Build history of the part. All positions in model axes, mm. Face numbers are marked on the shaded views. A direction names the side the tool comes from. Give positions to 0.01 mm unless a question says otherwise; leave off trailing zeros. Order: outer loops, then holes, each group sorted by start corner. A loop starts at its lowest first (then second) coordinate and runs counter-clockwise, first axis right, second up. Notation, with made-up numbers: (48, -38.75) -> (74, -38.75) arc R28 cw to (74, -17.75) -> close; hole circle Ø5 at (-26, 43). An arc over 180 degrees is marked (long way). One line per item, written item: value. Start each with the question number.
(1) Saw through at D-D on y = 4. Give the cut face in (x, z) (3 decimals).
(2) Saw through at A-A on y = -2. Give the cut face in (x, z) (3 decimals), plus the area to 3 significant figures.
(3) Saw through at B-B on y = 11. Give the cut face in (x, z) (3 decimals), plus the area to 3 significant figures.
(4) Two-plate mould, pull along X, no slides. Class the marked faces 1, 2 and 3: +X half, -X half, draft (parallel to the pull), parting line (faces both ways), or undercut.
(5) Saw through at C-C on x = -1.5. Give the cut face in (y, z) (3 decimals).
(6) Which spindle directions (+Z, -Z, +X, -X, +Y, -Y) get a long thin tool onto all of the face, cutting with end or side? Do the marked faces 4, 5, 6 and 7. Say none if no direction does.
(7) Pin check, flat tips, straight feed: pin 1 (1.3 mm diameter, centred on y = 23.5, z = 0.5, fed in from -X); pin 2 (3 mm diameter, centred on y = 18.5, z = 1.5, fed in from +X); pin 3 (3 mm diameter, centred on x = 13, z = 0, fed in from -Y); pin 4 (2.5 mm diameter, centred on x = -1, y = 11, fed in from +Z). Stop position of each tip, or through.
(8) Probe line 1 (X direction, y = -3.5, z = -1); line 2 (Z direction, x = 9.6, y = -6) (3 decimals); line 3 (Y direction, x = 13, z = 0). List the from-to ranges inside material, lowest first.
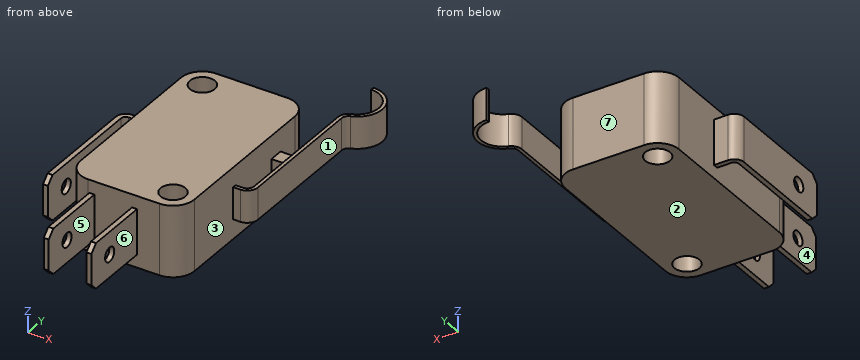
```python
from build123d import *

# Parameters (mm, degrees)
ESBO_O1_W             = 16
ESBO_O1_H             = 28
EXTRUS_O1_DEPTH       = 5
FILETE1_R             = 3
ESBO_O2_R             = 1.75
CORTE_EXTRUS_O1_DEPTH = 34.763886032
FLANGE_BASE1_START    = -2.25
FLANGE_BASE1_DEPTH    = 4.5
EXTRUS_O2_DEPTH       = 1.75
EXTRUS_O_FINA1_DEPTH  = 3.175
ESBO_O6_4_W           = 0.7
ESBO_O6_4_H           = 10
EXTRUS_O_FINA2_DEPTH  = 3.175
ESBO_O6_5_W           = 0.7
ESBO_O6_5_H           = 10
EXTRUS_O_FINA3_DEPTH  = 3.175
CHANFRO1_SIZE         = 1
ESBO_O7_R             = 1
CORTE_EXTRUS_O8_DEPTH = 3.35
ESBO_O7_6_R           = 1
CORTE_EXTRUS_O9_DEPTH = 47.597558949


# Read off the part's stored shape, not the designer's step: Flange-base1
with BuildPart() as part:
    # Esbo_o1 → Extrus_o1 (new, symmetric)
    with BuildSketch(Plane.XY):
        with Locations((8, 14)):
            Rectangle(ESBO_O1_W, ESBO_O1_H)
    extrude(amount=EXTRUS_O1_DEPTH, both=True)

    # Filete1
    filete1_edges = [part.edges().sort_by_distance(p)[0] for p in [
        (0, 28, 0),
        (16, 28, 0),
        (16, 0, 0),
        (0, 0, 0),
    ]]
    fillet(filete1_edges, radius=FILETE1_R)

    # Esbo_o2 → Corte-extrus_o1 (cut, through all)
    with BuildSketch(Plane.XY.offset(5)):
        with Locations((3, 25)):
            Circle(ESBO_O2_R)
        with Locations((13, 3)):
            Circle(ESBO_O2_R)
    extrude(amount=-CORTE_EXTRUS_O1_DEPTH, mode=Mode.SUBTRACT)



with BuildPart() as body_2:
    # Flange-base1 outline → Flange-base1 (new body)
    with BuildSketch(Plane.XY.offset(FLANGE_BASE1_START)):
        with BuildLine():
            ThreePointArc((19.166666667, 32.300168354), (21.449594959, 36.191856925), (18, 39.1))
            Line((18, 39.1), (18, 38.6))
            ThreePointArc((18, 38.6), (20.956795679, 36.107305936), (19, 32.771572875))
            ThreePointArc((19, 32.771572875), (18.275255129, 32.223384717), (18, 31.357359313))
            Line((18, 31.357359313), (18, 13))
            ThreePointArc((18, 13), (17.707106781, 12.292893219), (17, 12))
            Line((17, 12), (16, 12))
            Line((16, 12), (16, 11.5))
            Line((16, 11.5), (17, 11.5))
            ThreePointArc((17, 11.5), (18.060660172, 11.939339828), (18.5, 13))
            Line((18.5, 13), (18.5, 31.357359313))
            ThreePointArc((18.5, 31.357359313), (18.683503419, 31.934709582), (19.166666667, 32.300168354))
        make_face()
    extrude(amount=FLANGE_BASE1_DEPTH)


with BuildPart() as part_1:
    add(part.part)

    add(body_2.part)  # Extrus_o2 merges body 2
    # Esbo_o5 → Extrus_o2 (add, symmetric)
    with BuildSketch(Plane.XY):
        with BuildLine():
            Line((16, 21.874244368), (17.5, 21.874244368))
            ThreePointArc((17.5, 21.874244368), (17.853553391, 21.727797759), (18, 21.374244368))
            Line((18, 21.374244368), (18, 20.374244368))
            ThreePointArc((18, 20.374244368), (17.853553391, 20.020690978), (17.5, 19.874244368))
            Line((17.5, 19.874244368), (16, 19.874244368))
            Line((16, 19.874244368), (16, 21.874244368))
        make_face()
    extrude(amount=EXTRUS_O2_DEPTH, both=True)

    # Esbo_o6 → Extrus_o-Fina1 (add, symmetric)
    with BuildSketch(Plane.XY):
        with BuildLine():
            Line((0, 17.35), (-2, 17.35))
            ThreePointArc((-2, 17.35), (-2.954594155, 16.954594155), (-3.35, 16))
            Line((-3.35, 16), (-3.35, 0))
            Line((-3.35, 0), (-2.65, 0))
            Line((-2.65, 0), (-2.65, 16))
            ThreePointArc((-2.65, 16), (-2.459619408, 16.459619408), (-2, 16.65))
            Line((-2, 16.65), (0, 16.65))
            Line((0, 16.65), (0, 17.35))
        make_face()
    extrude(amount=EXTRUS_O_FINA1_DEPTH, both=True)

    # Esbo_o6_4 → Extrus_o-Fina2 (add, symmetric)
    with BuildSketch(Plane.XY):
        with Locations((3.526922814, -5)):
            Rectangle(ESBO_O6_4_W, ESBO_O6_4_H)
    extrude(amount=EXTRUS_O_FINA2_DEPTH, both=True)

    # Esbo_o6_5 → Extrus_o-Fina3 (add, symmetric)
    with BuildSketch(Plane.XY):
        with Locations((3.526922814, -5)):
            Rectangle(ESBO_O6_5_W, ESBO_O6_5_H)
        with BuildLine():
            Line((0, 17.35), (-2, 17.35))
            ThreePointArc((-2, 17.35), (-2.954594155, 16.954594155), (-3.35, 16))
            Line((-3.35, 16), (-3.35, 0))
            Line((-3.35, 0), (-2.65, 0))
            Line((-2.65, 0), (-2.65, 16))
            ThreePointArc((-2.65, 16), (-2.459619408, 16.459619408), (-2, 16.65))
            Line((-2, 16.65), (0, 16.65))
            Line((0, 16.65), (0, 17.35))
        make_face()
        with Locations((9.526922814, -5)):
            Rectangle(ESBO_O6_5_W, ESBO_O6_5_H)
    extrude(amount=EXTRUS_O_FINA3_DEPTH, both=True)

    # Chanfro1
    chanfro1_edges = [part_1.edges().sort_by_distance(p)[0] for p in [
        (-3, 0, -3.175),
        (3.526922814, -10, 3.175),
        (3.526922814, -10, -3.175),
        (9.526922814, -10, 3.175),
        (9.526922814, -10, -3.175),
        (-3, 0, 3.175),
    ]]
    chamfer(chanfro1_edges, length=CHANFRO1_SIZE)

    # Esbo_o7 → Corte-extrus_o8 (cut)
    with BuildSketch(Plane.ZY.offset(3.35)):
        with Locations(Location((0, 4, 0), (0, 0, 270))):
            Circle(ESBO_O7_R)
    extrude(amount=-CORTE_EXTRUS_O8_DEPTH, mode=Mode.SUBTRACT)

    # Esbo_o7_6 → Corte-extrus_o9 (cut, through all)
    with BuildSketch(Plane.ZY.offset(3.35)):
        with Locations(Location((0, -6, 0), (0, 0, 90))):
            Circle(ESBO_O7_6_R)
    extrude(amount=-CORTE_EXTRUS_O9_DEPTH, mode=Mode.SUBTRACT)


solid = part_1.part
```
Results below:
1. outline: (-3.35, -3.175) -> (-2.65, -3.175) -> (-2.65, -1) -> (-3.35, -1) -> close; (-3.35, 1) -> (-2.65, 1) -> (-2.65, 3.175) -> (-3.35, 3.175) -> close; (0, -5) -> (11.564, -5) -> (11.564, 5) -> (0, 5) -> close; (14.436, -5) -> (16, -5) -> (16, 5) -> (14.436, 5) -> close
2. outline: (3.177, -3.175) -> (3.877, -3.175) -> (3.877, 3.175) -> (3.177, 3.175) -> close; (9.177, -3.175) -> (9.877, -3.175) -> (9.877, 3.175) -> (9.177, 3.175) -> close
2. area: 8.89 mm²
3. outline: (-3.35, -3.175) -> (-2.65, -3.175) -> (-2.65, 3.175) -> (-3.35, 3.175) -> close; (0, -5) -> (16, -5) -> (16, 5) -> (0, 5) -> close
3. area: 164 mm²
4. face 1: +X half
4. face 2: draft
4. face 3: undercut
5. outline: (16.65, -3.175) -> (17.35, -3.175) -> (17.35, 3.175) -> (16.65, 3.175) -> close
6. face 4: +Z, -Z, -X, -Y
6. face 5: +Z, -Z, -Y
6. face 6: +Z, -Z, +X, -Y
6. face 7: +Z, -Z, -X, +Y
7. pin 1: stops at x = 0
7. pin 2: stops at x = 18.5
7. pin 3: stops at y = 0
7. pin 4: stops at z = 5
8. line 1: x = 3.18 to 3.88, 9.18 to 9.88
8. line 2: z = -3.175 to -1, 1 to 3.175
8. line 3: y = 0 to 1.25, 4.75 to 28
